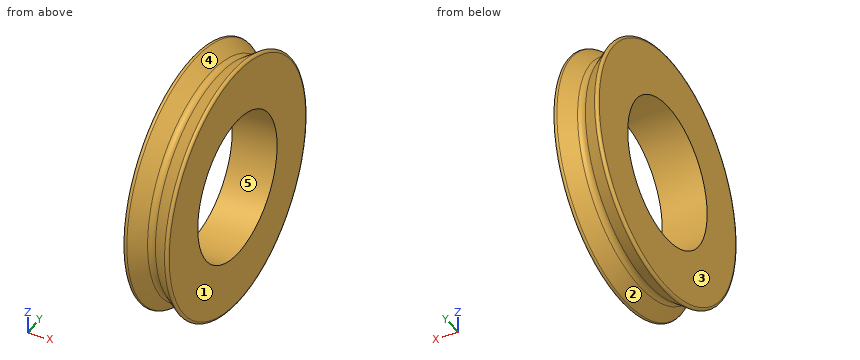
```python
from build123d import *


with BuildPart() as f1:
    # F0 (on Front) → F1 (revolve)
    with BuildSketch(Plane.XZ):
        with BuildLine():
            Line((2.089512, 13.857055), (0.437065, 12.7))
            ThreePointArc((0.437065, 12.7), (0, 12.562194), (-0.437065, 12.7))
            Line((-0.437065, 12.7), (-2.089512, 13.857055))
            ThreePointArc((-2.089512, 13.857055), (-2.352484, 13.874292), (-2.4892, 13.648991))
            Line((-2.4892, 13.648991), (-2.4892, 7.9375))
            Line((-2.4892, 7.9375), (0, 7.9375))
            Line((0, 7.9375), (2.4892, 7.9375))
            Line((2.4892, 7.9375), (2.4892, 13.648991))
            ThreePointArc((2.4892, 13.648991), (2.352484, 13.874292), (2.089512, 13.857055))
        make_face()
    revolve(axis=Axis((2.944905, 0, 0), (1, 0, 0)))


solid = f1.part
```
Geometry: final body of the model. Coordinates: model frame, mm. Face numbers are marked on the shaded views. A direction names the side the tool comes from. Round coordinates to 2 decimals unless told otherwise and drop trailing zeros. Order: outer loops, then holes, each group sorted by start corner. A loop starts at its lowest first (then second) coordinate and runs counter-clockwise, first axis right, second up. Notation, with made-up numbers: (71, 54) - (80, 54) arc R23 ccw to (80, 76) - close; hole circle Ø2 at (6.25, 7.5). An arc over 180 degrees is marked (long way). Use CSV: the item, a comma, the result in double quotes. Start each with the question number.
Q1. Section query A-A (y = 0). Return loops of the section in (x, z), and give its area (3 significant figures).
Q2. Mould query, pull axis Y, two halves, no side actions, for the marked faces 3, 4 and 5. Classes: +Y half, -Y half, draft (parallel to the pull), parting line (faces both ways), or undercut.
Q3. Access query for the marked faces 1 and 2. Directions: +Z, -Z, +X, -X, +Y, -Y. A direction counts if a zero-diameter tool reaches every point of the face in a straight line with its end or side. Return the directions, or none.
Q4. Section query C-C (x = -1.4). Return loops of the section in (y, z) (1 decimal).
Q5. Material intervals for line 1 along Z through (x, y) = (2.1, 0); line 2 along Z through (x, y) = (-0.5, 0); line 3 along Y through (x, z) = (1.05, 3), sorted ascending. Write a range as from..to.
Q6. First-contact query: pin 1 (2 mm diameter, centred on x = 0, z = 1, fed in from -Y); pin 2 (1.5 mm diameter, centred on x = 1, z = 1, fed in from +Y). Flat tips, straight axial feed; report the tip coordinate or a pass-through.
Result set:
1,outline,"(-2.49, -13.65) arc R0.25 ccw to (-2.09, -13.86) - (-0.44, -12.7) arc R0.76 cw to (0.44, -12.7) - (2.09, -13.86) arc R0.25 ccw to (2.49, -13.65) - (2.49, -7.94) - (-2.49, -7.94) - close; (-2.49, 7.94) - (2.49, 7.94) - (2.49, 13.65) arc R0.25 ccw to (2.09, 13.86) - (0.44, 12.7) arc R0.76 cw to (-0.44, 12.7) - (-2.09, 13.86) arc R0.25 ccw to (-2.49, 13.65) - close"
1,area,"52.9 mm2"
2,face 3,"draft"
2,face 4,"parting line"
2,face 5,"undercut"
3,face 1,"+Z, -Z, +X, +Y, -Y"
3,face 2,"none"
4,outline,"circle Ø26.7 at (0, 0); hole circle Ø15.9 at (0, 0)"
5,line 1,"z = -13.86..-7.94, 7.94..13.86"
5,line 2,"z = -12.74..-7.94, 7.94..12.74"
5,line 3,"y = -12.78..-7.35, 7.35..12.78"
6,pin 1,"stops at y = -13.06"
6,pin 2,"stops at y = 13.59"
